The listing builds one solid part. Answer for the finished solid, in the listing's coordinates (mm). A direction names the side the tool comes from. Coordinates: 2 decimals unless noted, no trailing zeros. Order: outer loops, then holes, each group sorted by start corner. A loop starts at its lowest first (then second) coordinate and runs counter-clockwise, first axis right, second up.
from build123d import *

# Parameters (mm, degrees)
SKIZZE1_W                       = 35
SKIZZE1_H                       = 75
AUFSATZ_LINEAR_AUSTRAGEN1_DEPTH = 1.5
SKIZZE2_W                       = 11.63
SKIZZE2_H                       = 5
SKIZZE2_W_2                     = 11.62
SKIZZE2_W_3                     = 1.75
SCHNITT_LINEAR_AUSTRAGEN1_DEPTH = 1.5
SCHNITT_LINEAR_AUSTRAGEN7_DEPTH = 20


with BuildPart() as part:
    # Skizze1 → Aufsatz-Linear austragen1 (new body)
    with BuildSketch(Plane.XY):
        with Locations((17.5, 37.5)):
            Rectangle(SKIZZE1_W, SKIZZE1_H)
    extrude(amount=AUFSATZ_LINEAR_AUSTRAGEN1_DEPTH)

    # Skizze2 → Schnitt-Linear austragen1 (cut)
    with BuildSketch(Plane.XY.offset(1.5)):
        with Locations((5.815, 2.5)):
            Rectangle(SKIZZE2_W, SKIZZE2_H)
        with Locations((29.19, 2.5)):
            Rectangle(SKIZZE2_W_2, SKIZZE2_H)
        with Locations((17.505, 2.5)):
            Rectangle(SKIZZE2_W_3, SKIZZE2_H)
    extrude(amount=-SCHNITT_LINEAR_AUSTRAGEN1_DEPTH, mode=Mode.SUBTRACT)

    # Skizze12 → Schnitt-Linear austragen7 (cut)
    with BuildSketch(Plane.XY.offset(1.5)):
        Polygon((6.459240655, 64.5), (28.25, 64.5), (28.25, 63.5), (8.976723544, 17), (7.894229713, 17), (27.167506169, 63.5), (6.459240655, 63.5), align=None)
    extrude(amount=-SCHNITT_LINEAR_AUSTRAGEN7_DEPTH, mode=Mode.SUBTRACT)


solid = part.part
1) A tool of negligible diameter and unlimited length cuts with its end or side. For faces 4 (the face through (17, 63.5, 1)), 5 (the face through (29, 5, 1)), 6 (the face through (17, 5, 1)), from which of +Z, -Z, +X, -X, +Y, -Y can it reach the whole face along a straight path? Write none if from no direction.
2) Section C-C (y = 40.5) is taken. Give the vertices of the cut face in (x, z), then the cut area to 3 significant figures.
3) Determine the mould class of faces 1 (the face through (17, 64.5, 1)), 2 (the face through (0, 40, 1)), 3 (the face through (17, 46, 0)) for opening direction X: released by +X, released by -X, zero draft, split by the parting line, or undercut.
4) Section D-D (x = 30) is taken. Give the vertices of the cut face in (y, z), then the cut area to 3 significant figures.
5) Section B-B (x = 25) is taken. Give the vertices of the cut face in (y, z), then the cut area to 3 significant figures.
6) Section A-A (z = 0.7) is taken. Give the vertices of the cut face in (x, y), then the cut area to 3 significant figures.
7) Consider L1, parallel to Y at x = 13, z = 0.3; L2, parallel to Y at x = 10.5, z = 0.35; L3, parallel to Y at x = 3, z = 1.35. Determine where each line is inside the solid, lowest interval first.
Filled sheet:
1. face 4: +Z, -Z
1. face 5: +Z, -Z, +X, -Y
1. face 6: +Z, -Z, -Y
2. outline: (0, 0) - (17.63, 0) - (17.63, 1.5) - (0, 1.5) - close; (18.72, 0) - (35, 0) - (35, 1.5) - (18.72, 1.5) - close
2. area: 50.9 mm2
3. face 1: undercut
3. face 2: released by -X
3. face 3: zero draft
4. outline: (5, 0) - (75, 0) - (75, 1.5) - (5, 1.5) - close
4. area: 105 mm2
5. outline: (5, 0) - (55.66, 0) - (55.66, 1.5) - (5, 1.5) - close; (58.27, 0) - (63.5, 0) - (63.5, 1.5) - (58.27, 1.5) - close; (64.5, 0) - (75, 0) - (75, 1.5) - (64.5, 1.5) - close
5. area: 99.6 mm2
6. outline: (0, 5) - (11.63, 5) - (11.63, 0) - (16.63, 0) - (16.63, 5) - (18.38, 5) - (18.38, 0) - (23.38, 0) - (23.38, 5) - (35, 5) - (35, 75) - (0, 75) - close; hole (6.46, 63.5) - (27.17, 63.5) - (7.89, 17) - (8.98, 17) - (28.25, 63.5) - (28.25, 64.5) - (6.46, 64.5) - close
6. area: 2,430 mm2
7. L1: y = 0 to 26.71, 29.32 to 63.5, 64.5 to 75
7. L2: y = 5 to 20.68, 23.29 to 63.5, 64.5 to 75
7. L3: y = 5 to 75
